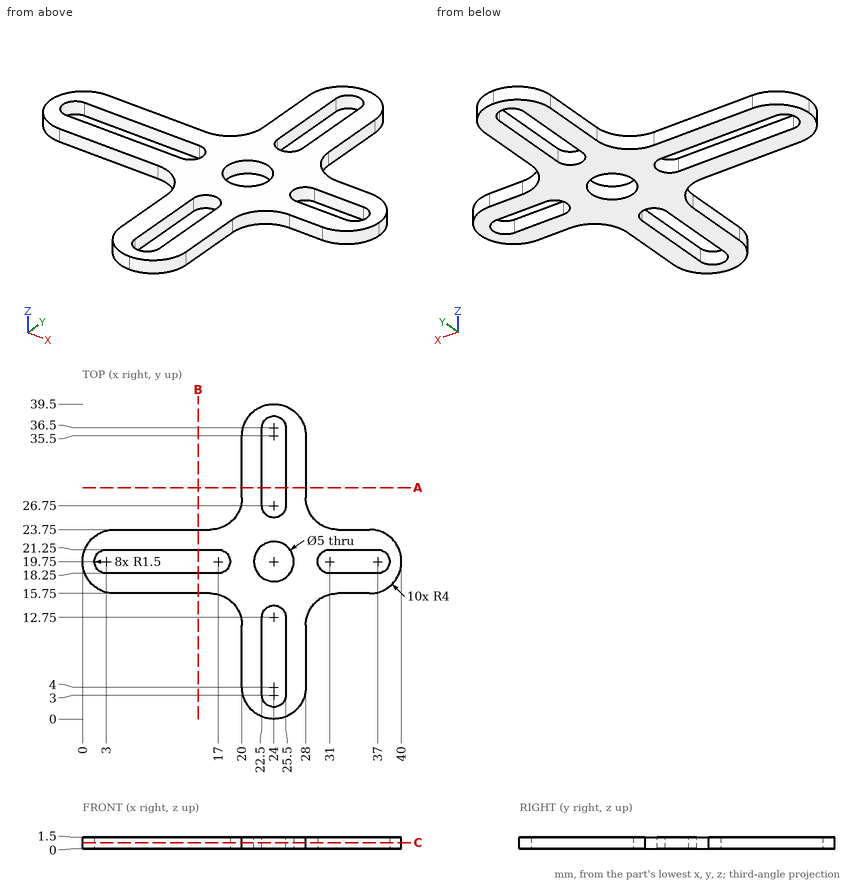
For this review, use the dimensioned drawing (mm, ordinates from the lowest corner) and the shaded views. Coordinates: 2 decimals unless noted, no trailing zeros. Order: outer loops, then holes, each group sorted by start corner. A loop starts at its lowest first (then second) coordinate and runs counter-clockwise, first axis right, second up. Notation, with made-up numbers: M 33,71.5 L 44,71.5 A16 ccw 44,86.5 Z; hole C 52,53 d6. An arc over 180 degrees is marked long. Answer as a JSON object with one key per item and string values. Group by question number.
1) For pin 1 (0.8 mm diameter, centred on y = 8, z = 1, fed in from +X); pin 2 (0.8 mm diameter, centred on y = 6.5, z = 1, fed in from -X); pin 3 (0.8 mm diameter, centred on x = 11.5, z = 0.5, fed in from -Y); pin 4 (5 mm diameter, centred on x = 23, y = 7, fed in from -Z), all flat-tipped, find the tip position at first contact; note any pin that passes through.
2) Wall thickness on L1, parallel to Y at x = 24, z = 1.2; L2, parallel to X at y = 7, z = 0.1; L3, parallel to Y at x = 9, z = 1.4: over which ranges is each line inside the solid? List them lowest first.
3) Add section A-A, the plane y = 29. Write out the cut boundary in (x, z).
4) Add section B-B, the plane x = 14.5. Write out the cut boundary in (y, z), then the cut area to 3 significant figures.
5) Add section C-C, the plane z = 0.8. Count the separate pieces of the cut face and the enclosed holes in it, then the cut area to 3 significant figures.
Computed values:
{
 "1": {"pin 1": "stops at x = 28", "pin 2": "stops at x = 20", "pin 3": "stops at y = 15.75", "pin 4": "stops at z = 0"},
 "2": {"L1": "y = 0 to 1.5, 14.25 to 17.25, 22.25 to 25.25, 38 to 39.5", "L2": "x = 20 to 22.5, 25.5 to 28", "L3": "y = 15.75 to 18.25, 21.25 to 23.75"},
 "3": {"outline": "M 20,0 L 22.5,0 L 22.5,1.5 L 20,1.5 Z; M 25.5,0 L 28,0 L 28,1.5 L 25.5,1.5 Z"},
 "4": {"outline": "M 15.75,0 L 18.25,0 L 18.25,1.5 L 15.75,1.5 Z; M 21.25,0 L 23.75,0 L 23.75,1.5 L 21.25,1.5 Z", "area": "7.50 mm^2"},
 "5": {"separate pieces": "1", "enclosed holes": "5", "area": "392 mm^2"}
}
